Input: part model. Units: mm. Frame: model coordinates. A direction names the side the tool comes from. Give positions to 0.01 mm unless a question says otherwise; leave off trailing zeros. Write each loop counter-clockwise with the first axis right and the second up, starting at its lowest first coordinate (ties: lowest second). Pieces come first, ordered by that corner, then holes. Notation, with made-up numbers: (58.5, -30) - (62.5, -30) arc R35 ccw to (62.5, 2) - close; hole circle Ø4 at (-22, 4.25). An arc over 180 degrees is marked (long way). Answer as a JSON object with one key per item and string values. Group by question number.
Autodesk Inventor part; units mm, degrees
ref_plane "Plano de trabajo1" through (75, 0, 0) normal (1, 0, 0) x (0, 0, -1)
ref_plane "Plano de trabajo2" through (150, 25, 68) normal (0, 0, 1) x (1, 0, 0)
ref_plane "Plano de trabajo3" through (75, 0, 0) normal (1, 0, 0) x (0, 0, -1)
sketch "Boceto1" plane through (0, 0, 0) normal (0, 0, 1) x (1, 0, 0)
  line L0 (0, 0) -> (150, 0)
  line L1 (150, 0) -> (150, 150)
  line L2 (150, 150) -> (0, 150)
  line L3 (0, 150) -> (0, 0)
  line L4 (5, 145) -> (145, 145)
  line L5 (145, 145) -> (145, 5)
  line L6 (145, 5) -> (5, 5)
  line L7 (5, 5) -> (5, 145)
  dimension "d0" = 150
  dimension "d1" = 150
  dimension "d2" = 5
extrude "Extrusión1" add sketch "Boceto1" along normal blind 150
sketch "Boceto2" plane through (150, 0, 0) normal (1, 0, 0) x (0, 0, -1)
  line L0 (-150, 0) -> (-150, 150)
  line L1 (-150, 75) -> (-190, 75) construction
  line L2 (-190, 75) -> (-150, 150)
  line L3 (0, 0) -> (-150, 0) construction
  line L4 (-150, 0) -> (-190, 75)
  dimension "d5" = 40
extrude "Extrusión2" add sketch "Boceto2" against normal blind 5
ref_plane "Plano de trabajo1" through (75, 0, 0) normal (1, 0, 0) x (0, 0, -1)
mirror "Simetría1" about plane through (75, 0, 0) normal (1, 0, 0) of "Extrusión2"
sketch "Boceto3" plane through (0, 150, 0) normal (0, 1, 0) x (1, 0, 0)
  line L0 (105, -60) -> (45, -60)
  line L1 (45, -60) -> (45, -95)
  line L2 (60, -110) -> (90, -110)
  line L3 (105, -95) -> (105, -60)
  line L4 (150, 0) -> (0, 0)
  line L5 (145, -150) -> (5, -150)
  arc A0 (90, -110) -> (105, -95) centre (90, -95) ccw
  arc A1 (45, -95) -> (60, -110) centre (60, -95) ccw
  point P0 (45, -110)
  point P1 (105, -110)
  point P2 (75, -60)
  point P3 (75, 0)
  dimension "d8" = 60
  dimension "d9" = 50
  dimension "d10" = 40
  dimension "d11" = 15
extrude "Extrusión3" cut sketch "Boceto3" against normal through all
sketch "Boceto4" plane through (150, 0, 0) normal (1, 0, 0) x (0, 0, -1)
  line L0 (-13, 20) -> (-123, 20)
  line L1 (-128, 25) -> (-128, 75)
  line L2 (-123, 80) -> (-13, 80)
  line L3 (-8, 75) -> (-8, 25)
  line L4 (0, 0) -> (0, 150)
  line L5 (0, 0) -> (-150, 0)
  arc A0 (-123, 80) -> (-128, 75) centre (-123, 75) ccw
  arc A1 (-8, 75) -> (-13, 80) centre (-13, 75) ccw
  arc A2 (-13, 20) -> (-8, 25) centre (-13, 25) ccw
  arc A3 (-128, 25) -> (-123, 20) centre (-123, 25) ccw
  point P0 (-128, 80)
  point P1 (-128, 20)
  point P2 (-8, 80)
  dimension "d14" = 120
  dimension "d15" = 60
  dimension "d16" = 8
  dimension "d17" = 20
  dimension "d18" = 5
extrude "Extrusión4" cut sketch "Boceto4" against normal up to surface (5 mm away)
sketch "Boceto5" plane through (0, 0, 0) normal (-1, 0, 0) x (0, 0, 1)
  line L0 (65, 125) -> (115, 125)
  line L1 (120, 120) -> (120, 30)
  line L2 (115, 25) -> (65, 25)
  line L3 (60, 30) -> (60, 120)
  line L4 (0, 150) -> (0, 0)
  arc A0 (120, 120) -> (115, 125) centre (115, 120) ccw
  arc A1 (115, 25) -> (120, 30) centre (115, 30) ccw
  arc A2 (65, 125) -> (60, 120) centre (65, 120) ccw
  arc A3 (60, 30) -> (65, 25) centre (65, 30) ccw
  point P0 (60, 150)
  point P1 (120, 25)
  point P2 (120, 125)
  point P3 (60, 25)
  point P4 (60, 75)
  point P5 (0, 75)
  dimension "d21" = 60
  dimension "d22" = 100
  dimension "d23" = 60
  dimension "d24" = 5
extrude "Extrusión5" cut sketch "Boceto5" against normal blind 10
sketch "Boceto6" plane through (150, 0, 0) normal (1, 0, 0) x (0, 0, -1)
  line L0 (-190, 75) -> (-150, 0)
  line L1 (-150, 150) -> (-190, 75)
  line L2 (-154.4118, 152.3529) -> (-195.6667, 75)
  line L3 (-195.6667, 75) -> (-154.4118, -2.3529)
  line L4 (-154.4118, 152.3529) -> (-144.4118, 152.3529)
  line L5 (-144.4118, 152.3529) -> (-144.4118, 150)
  line L6 (-154.4118, -2.3529) -> (-144.4118, -2.3529)
  line L7 (-144.4118, -2.3529) -> (-144.4118, 0)
  line L8 (0, 0) -> (-150, 0)
  line L9 (0, 150) -> (-150, 150)
  dimension "d27" = 5
  dimension "d28" = 10
extrude "Extrusión6" add sketch "Boceto6" along normal blind 10 and the other way blind 160
fillet "Empalme1" radius 5 3 edges at (75, 152.3529, 154.4118) (75, 75, 195.6667) (75, -2.3529, 154.4118)
sketch "Boceto7" plane through (150, 25, 8) normal (0, 0, 1) x (1, 0, 0)
  circle A0 centre (-2.5, 2.5) radius 1.25
  line L0 (0, 50) -> (0, 0)
  line L1 (0, 0) -> (-5, 0)
  point P0 (-150, -25)
  point P1 (-2.5, 0)
  dimension "d34" = 2.5
  dimension "d35" = 2.5
  dimension "d36" = 2.5
extrude "Extrusión7" cut sketch "Boceto7" against normal blind 3
ref_plane "Plano de trabajo2" through (150, 25, 68) normal (0, 0, 1) x (1, 0, 0)
mirror "Simetría2" about plane through (150, 25, 68) normal (0, 0, 1) of "Extrusión7"
sketch "Boceto8" plane through (160, 0, 0) normal (1, 0, 0) x (0, 0, -1)
  arc A0 (-155.8235, 0.2941) -> (-151.4118, -2.3529) centre (-151.4118, 2.6471) ccw
  line L0 (-151.4118, -2.3529) -> (-144.4118, -2.3529)
  line L1 (-144.4118, -2.3529) -> (-144.4118, 0)
  line L2 (-144.4118, 0) -> (-150, 0)
  line L3 (-150, 0) -> (-190, 75)
  line L4 (-190, 75) -> (-150, 150)
  line L5 (-150, 150) -> (-144.4118, 150)
  line L6 (-144.4118, 150) -> (-144.4118, 152.3529)
  line L7 (-144.4118, 152.3529) -> (-151.4118, 152.3529)
  arc A1 (-151.4118, 152.3529) -> (-155.8235, 149.7059) centre (-151.4118, 147.3529) ccw
  line L8 (-155.8235, 149.7059) -> (-194.4118, 77.3529)
  arc A2 (-194.4118, 77.3529) -> (-194.4118, 72.6471) centre (-190, 75) ccw
  line L9 (-194.4118, 72.6471) -> (-155.8235, 0.2941)
  point P0 (0, 0)
extrude "Extrusión8" cut sketch "Boceto8" against normal through all
sketch "Boceto9" plane through (145, 0, 150) normal (0, -0.4705882, 0.8823529) x (1, 0, 0)
  circle A0 centre (2.5, 2.5) radius 1.5
  line L0 (5, 85) -> (5, 0)
  line L1 (5, 0) -> (0, 0)
  point P0 (-145, -70.5882)
  dimension "d41" = 3
  dimension "d42" = 2.5
  dimension "d43" = 2.5
extrude "Extrusión9" cut sketch "Boceto9" against normal blind 5
ref_plane "Plano de trabajo3" through (75, 0, 0) normal (1, 0, 0) x (0, 0, -1)
ref_plane "Plano de trabajo4" through (0, 75, 0) normal (0, -1, 0) x (1, 0, 0)
mirror "Simetría3" about plane through (75, 0, 0) normal (1, 0, 0) of "Extrusión9"
mirror "Simetría4" about plane through (0, 75, 0) normal (0, -1, 0) of "Extrusión8", "Extrusión9", "Simetría3"
sketch "Boceto10" plane through (0, 0, 0) normal (-1, 0, 0) x (0, 0, 1)
  line L0 (190, 75) -> (150, 0)
  line L1 (0, 0) -> (150, 0)
  arc A0 (115, 25) -> (120, 30) centre (115, 30) ccw
  line L2 (115, 25) -> (65, 25)
  arc A1 (60, 30) -> (65, 25) centre (65, 30) ccw
  line L3 (60, 30) -> (60, 120)
  arc A2 (65, 125) -> (60, 120) centre (65, 120) ccw
  line L4 (65, 125) -> (115, 125)
  arc A3 (120, 120) -> (115, 125) centre (115, 120) ccw
  line L5 (120, 120) -> (120, 30)
  line L6 (0, 150) -> (0, 0)
  line L7 (0, 0) -> (150, 0)
  line L8 (190, 75) -> (150, 0)
  line L9 (150, 150) -> (190, 75)
  line L10 (0, 150) -> (150, 150)
  line L11 (0, 150) -> (150, 150)
  line L12 (150, 150) -> (190, 75)
extrude "Extrusión10" cut sketch "Boceto10" against normal up to surface (145 mm away) contours L0 L1 L6 L10 L9 | L2 A1 L3 A2 L4 A3 L5 A0
sketch "Boceto11" plane through (145, 0, 0) normal (-1, 0, 0) x (0, 0, 1)
  circle A0 centre (147.5, 2.5) radius 1.5
  line L0 (0, 0) -> (150, 0)
  line L1 (75, 0) -> (75, 157.0348) construction
  line L2 (0, 0) -> (0, 150)
  line L3 (0, 75) -> (163.5467, 75) construction
  circle A1 centre (147.5, 147.5) radius 1.5
  circle A2 centre (2.5, 2.5) radius 1.5
  circle A3 centre (2.5, 147.5) radius 1.5
  dimension "d48" = 2.5
  dimension "d49" = 3
  dimension "d50" = 2.5
extrude "Extrusión11" add sketch "Boceto11" along normal blind 5
properties part number "CasaJugueteAPM" material "Plástico ABS"
1) Cut plane B-B on x = 142.25. Return the cut outline in (y, z), and give its area (3 significant figures).
2) Pin query (flat end, axial travel): P1, Ø5.5, axis at x = 148.5, y = 39.5, coming from the +Z side; P2, Ø1.5, axis at x = 147.5, y = 58.5, coming from the -Z side; P3, Ø2, axis at x = 147, y = 27.5, coming from the +Z side; P4, Ø3, axis at x = 147.5, y = 27.5, coming from the +Z side. Return the tip coordinate at first contact, or that it passes through.
3) Mould query, pull axis X, two halves, no side actions, for faces 1 (the face through (148.886, 146.127, 149.271)), 2 (the face through (148, 21, 10)), 3 (the face through (150, 91, 94)). Classes: +X half, -X half, draft (parallel to the pull), parting line (faces both ways), or undercut.
4) Cut plane D-D on y = 119. Return the cut outline in (x, z), and give its area (3 significant figures).
5) Cut plane C-C on z = 162. Return the cut outline in (x, y), and give its area (3 significant figures).
6) Line query: line 1 along Y through (x, z) = (147.5, 7); line 2 along Y through (x, z) = (147, 80.5); line 3 along Z through (x, y) = (147, 44). Output: solid intervals per line, ascending. Write a range as from..to.
7) Reachability of faces 4 (the face through (148.886, 2.859, 148.73)), 5 (the face through (148, 22, 127)) from +Z, -Z, +X, -X, +Y, -Y: full face, straight path, thin tool, end or side. Return the list, or none.
8) Cut plane A-A on z = 119. Return the cut outline in (x, y).
Filled in:
{
 "1": {"outline": "circle Ø3 at (2.5, 2.5); circle Ø3 at (2.5, 147.5); circle Ø3 at (147.5, 2.5); circle Ø3 at (147.5, 147.5)", "area": "28.3 mm²"},
 "2": {"P1": "stops at z = 172.53", "P2": "stops at z = 0", "P3": "stops at z = 165.2", "P4": "stops at z = 165.47"},
 "3": {"face 1": "undercut", "face 2": "draft", "face 3": "+X half"},
 "4": {"outline": "(145, 0) - (150, 0) - (150, 166.53) - (145, 166.53) - close", "area": "833 mm²"},
 "5": {"outline": "(145, 22.5) - (150, 22.5) - (150, 127.5) - (145, 127.5) - close", "area": "525 mm²"},
 "6": {"line 1": "y = 0..26.25, 28.75..150", "line 2": "y = 0..20, 80..150", "line 3": "z = 0..8, 128..173.47"},
 "7": {"face 4": "none", "face 5": "+X, -X"},
 "8": {"outline": "(145, 0) - (150, 0) - (150, 20) - (145, 20) - close; (145, 80) - (150, 80) - (150, 150) - (145, 150) - close"}
}
